Part print with two shaded views. Sizes in mm from the minimum x, y, z corner. Coordinates: 2 decimals unless noted, no trailing zeros. Write each loop counter-clockwise with the first axis right and the second up, starting at its lowest first coordinate (ties: lowest second). Pieces come first, ordered by that corner, then holes. Notation, with made-up numbers: M 53.25,85.5 L 105.25,85.5 A14 ccw 105.25,96.5 Z; hole C 17.5,67 d5. An arc over 180 degrees is marked long. Use CSV: the item, a comma, the result in double quotes. Start each with the question number.
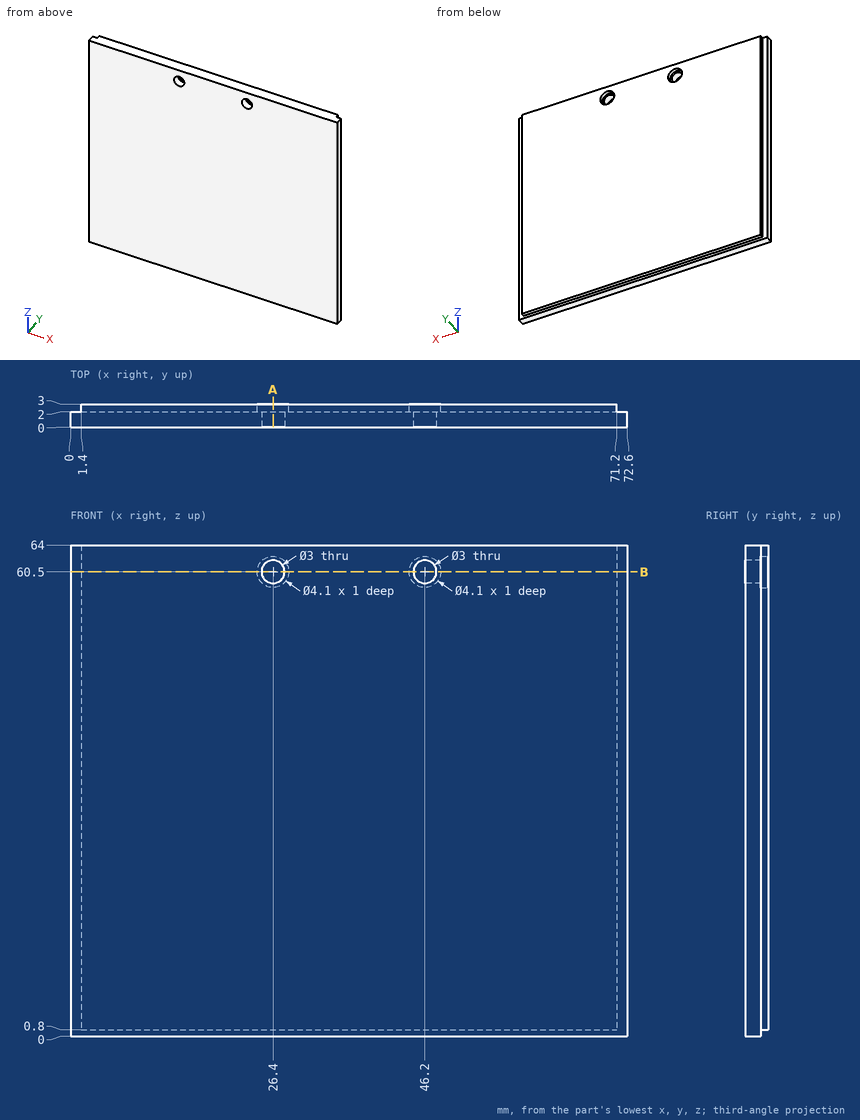
1. Drill centre lines: line 1 along X through (y, z) = (2.25, 60.5); line 2 along X through (y, z) = (1.3, 60.5); line 3 along Z through (x, y) = (46.2, 1.35). Where is each one in solid material? Low to high. Write a range as from..to.
2. Flat gauge pins, fed straight in: pin 1 (0.5 mm diameter, centred on y = 2.5, z = 31.5, fed in from -X); pin 2 (3.5 mm diameter, centred on x = 46.5, z = 61, fed in from +Y); pin 3 (0.8 mm diameter, centred on y = 2.5, z = 43.5, fed in from +X). Where does each tip first touch, or does it go through?
3. Slice it at A-A (x = 26.4). List the corners of the cut face in (y, z), and give its area (3 significant figures).
4. Slice it at B-B (z = 60.5). List the corners of the cut face in (x, y).
Established:
1,line 1,"x = 1.4..24.35, 28.45..44.15, 48.25..71.2"
1,line 2,"x = 0..24.9, 27.9..44.7, 47.7..72.6"
1,line 3,"z = 0..59, 62..64"
2,pin 1,"stops at x = 1.4"
2,pin 2,"stops at y = 3"
2,pin 3,"stops at x = 71.2"
3,outline,"M 0,0 L 2,0 L 2,0.8 L 3,0.8 L 3,58.45 L 2,58.45 L 2,59 L 0,59 Z; M 0,62 L 2,62 L 2,62.55 L 3,62.55 L 3,64 L 0,64 Z"
3,area,"181 mm2"
4,outline,"M 0,0 L 24.9,0 L 24.9,2 L 24.35,2 L 24.35,3 L 1.4,3 L 1.4,2 L 0,2 Z; M 27.9,0 L 44.7,0 L 44.7,2 L 44.15,2 L 44.15,3 L 28.45,3 L 28.45,2 L 27.9,2 Z; M 47.7,0 L 72.6,0 L 72.6,2 L 71.2,2 L 71.2,3 L 48.25,3 L 48.25,2 L 47.7,2 Z"
